The model under review builds one solid part; all positions refer to its coordinate system, in mm. Coordinates: 2 decimals unless noted, no trailing zeros. Loops run counter-clockwise (first coordinate to the right, second up) from the corner with the lowest first, then second, coordinate; pieces in that order, holes last. Notation, with made-up numbers: (30.25, 85.5) - (61.25, 85.5) arc R28 cw to (61.25, 108.5) - close; hole circle Ø8 at (14, 45.25). An arc over 180 degrees is marked (long way). One line per item, written item: value. Start each with the question number.
1. We need section C-C, the plane x = 15.5. Give the boundary of the cut face in (y, z), then the cut area to 3 significant figures.
2. To check wall thickness, follow line 1 (X direction, y = -15.5, z = -1.75); line 2 (Y direction, x = 15.5, z = -1.25); line 3 (X direction, y = 0, z = -3.2). State the ranges of each line that lie inside material, in increasing order.
3. We need section D-D, the plane z = -3. Give the boundary of the cut face in (x, y).
4. Insertion check: P1, Ø3.5, axis at x = -15.5, y = -15.5, coming from the +Z side. The pin has a flat end and moves straight along its axis. Give the tip position at first contact, or say it passes through.
5. We need section B-B, the plane x = 0. Give the boundary of the cut face in (y, z).
6. We need section A-A, the plane y = 15.5. Give the boundary of the cut face in (x, z).
7. Mouldability with a two-part tool opening along X and no side actions: class faces 1 (the face through (-17.483, -15.24, -2.535)), 2 (the face through (50, 0, -2)), 3 (the face through (-0.7, 11.5, -5)) as +X half, -X half, draft (parallel to the pull), parting line (faces both ways), or undercut.
Autodesk Inventor part; units mm, degrees
ref_plane "YZ Plane" through (0, 0, 0) normal (1, 0, 0) x (0, 1, 0)
ref_plane "XZ Plane" through (0, 0, 0) normal (0, 1, 0) x (-1, 0, 0)
ref_plane "XY Plane" through (0, 0, 0) normal (0, 0, 1) x (1, 0, 0)
sketch "Block1" plane through (0, 0, 0) normal (0, 0, 1) x (1, 0, 0)
  line L0 (-30.1, 34.1) -> (-9.9, 34.1)
  line L1 (-9.9, 34.1) -> (-9.9, 25.1)
  line L2 (-9.9, 25.1) -> (9.9, 25.1)
  line L3 (9.9, 25.1) -> (9.9, 34.1)
  line L4 (9.9, 34.1) -> (30.1, 34.1)
  line L5 (30.1, 34.1) -> (30.1, 25.1)
  line L6 (30.1, 25.1) -> (50.1, 25.1)
  line L7 (50.1, 25.1) -> (50.1, 16.5667)
  line L8 (50.1, 16.5667) -> (41.1, 16.5667)
  line L9 (41.1, 16.5667) -> (41.1, 6.7667)
  line L10 (41.1, 6.7667) -> (50.1, 6.7667)
  line L11 (50.1, 6.7667) -> (50.1, -6.7667)
  line L12 (50.1, -6.7667) -> (41.1, -6.7667)
  line L13 (41.1, -6.7667) -> (41.1, -16.5667)
  line L14 (41.1, -16.5667) -> (50.1, -16.5667)
  line L15 (50.1, -16.5667) -> (50.1, -25.1)
  line L16 (50.1, -25.1) -> (30.1, -25.1)
  line L17 (30.1, -25.1) -> (30.1, -34.1)
  line L18 (30.1, -34.1) -> (9.9, -34.1)
  line L19 (9.9, -34.1) -> (9.9, -25.1)
  line L20 (9.9, -25.1) -> (-9.9, -25.1)
  line L21 (-9.9, -25.1) -> (-9.9, -34.1)
  line L22 (-9.9, -34.1) -> (-30.1, -34.1)
  line L23 (-30.1, -34.1) -> (-30.1, -25.1)
  line L24 (-30.1, -25.1) -> (-50.1, -25.1)
  line L25 (-50.1, -25.1) -> (-50.1, -16.5667)
  line L26 (-50.1, -16.5667) -> (-41.1, -16.5667)
  line L27 (-41.1, -16.5667) -> (-41.1, -6.7667)
  line L28 (-41.1, -6.7667) -> (-50.1, -6.7667)
  line L29 (-50.1, -6.7667) -> (-50.1, 6.7667)
  line L30 (-50.1, 6.7667) -> (-41.1, 6.7667)
  line L31 (-41.1, 6.7667) -> (-41.1, 16.5667)
  line L32 (-41.1, 16.5667) -> (-50.1, 16.5667)
  line L33 (-50.1, 16.5667) -> (-50.1, 25.1)
  line L34 (-50.1, 25.1) -> (-30.1, 25.1)
  line L35 (-30.1, 25.1) -> (-30.1, 34.1)
  circle A0 centre (-30, 0) radius 4.6
  circle A1 centre (-15.5, 15.5) radius 2.1
  circle A2 centre (-15.5, -15.5) radius 2.1
  circle A3 centre (0, 0) radius 11.1
  circle A4 centre (15.5, 15.5) radius 2.1
  circle A5 centre (30, 0) radius 4.6
  circle A6 centre (15.5, -15.5) radius 2.1
  point P0 (0, 0)
sketch "Block2" plane through (0, 0, 0) normal (0, 0, 1) x (1, 0, 0)
  line L0 (9.8, 34.2) -> (30.2, 34.2)
  line L1 (30.2, 34.2) -> (30.2, 25.2)
  line L2 (30.2, 25.2) -> (50.2, 25.2)
  line L3 (50.2, 25.2) -> (50.2, 16.4667)
  line L4 (50.2, 16.4667) -> (41.2, 16.4667)
  line L5 (41.2, 16.4667) -> (41.2, 6.8667)
  line L6 (41.2, 6.8667) -> (50.2, 6.8667)
  line L7 (50.2, 6.8667) -> (50.2, -6.8667)
  line L8 (50.2, -6.8667) -> (41.2, -6.8667)
  line L9 (41.2, -6.8667) -> (41.2, -16.4667)
  line L10 (41.2, -16.4667) -> (50.2, -16.4667)
  line L11 (50.2, -16.4667) -> (50.2, -25.2)
  line L12 (50.2, -25.2) -> (30.2, -25.2)
  line L13 (30.2, -25.2) -> (30.2, -34.2)
  line L14 (30.2, -34.2) -> (9.8, -34.2)
  line L15 (9.8, -34.2) -> (9.8, -25.2)
  line L16 (9.8, -25.2) -> (-9.8, -25.2)
  line L17 (-9.8, -25.2) -> (-9.8, -34.2)
  line L18 (-9.8, -34.2) -> (-30.2, -34.2)
  line L19 (-30.2, -34.2) -> (-30.2, -25.2)
  line L20 (-30.2, -25.2) -> (-50.2, -25.2)
  line L21 (-50.2, -25.2) -> (-50.2, -16.4667)
  line L22 (-50.2, -16.4667) -> (-41.2, -16.4667)
  line L23 (-41.2, -16.4667) -> (-41.2, -6.8667)
  line L24 (-41.2, -6.8667) -> (-50.2, -6.8667)
  line L25 (-50.2, -6.8667) -> (-50.2, 6.8667)
  line L26 (-50.2, 6.8667) -> (-41.2, 6.8667)
  line L27 (-41.2, 6.8667) -> (-41.2, 16.4667)
  line L28 (-41.2, 16.4667) -> (-50.2, 16.4667)
  line L29 (-50.2, 16.4667) -> (-50.2, 25.2)
  line L30 (-50.2, 25.2) -> (-30.2, 25.2)
  line L31 (-30.2, 25.2) -> (-30.2, 34.2)
  line L32 (-30.2, 34.2) -> (-9.8, 34.2)
  line L33 (-9.8, 34.2) -> (-9.8, 25.2)
  line L34 (-9.8, 25.2) -> (9.8, 25.2)
  line L35 (9.8, 25.2) -> (9.8, 34.2)
  circle A0 centre (-15.5, 15.5) radius 2.2
  circle A1 centre (15.5, 15.5) radius 2.2
  circle A2 centre (30, 0) radius 4.7
  circle A3 centre (15.5, -15.5) radius 2.2
  circle A4 centre (-15.5, -15.5) radius 2.2
  circle A5 centre (-30, 0) radius 4.7
  circle A6 centre (0, 0) radius 11.2
  point P0 (0, 0)
sketch "Block3" plane through (0, 0, 0) normal (0, 0, 1) x (1, 0, 0)
  line L0 (9.9, 34.1) -> (30.1, 34.1)
  line L1 (30.1, 34.1) -> (30.1, 25.1)
  line L2 (30.1, 25.1) -> (50.1, 25.1)
  line L3 (50.1, 25.1) -> (50.1, 16.5667)
  line L4 (50.1, 16.5667) -> (41.1, 16.5667)
  line L5 (41.1, 16.5667) -> (41.1, 6.7667)
  line L6 (41.1, 6.7667) -> (50.1, 6.7667)
  line L7 (50.1, 6.7667) -> (50.1, -6.7667)
  line L8 (50.1, -6.7667) -> (41.1, -6.7667)
  line L9 (41.1, -6.7667) -> (41.1, -16.5667)
  line L10 (41.1, -16.5667) -> (50.1, -16.5667)
  line L11 (50.1, -16.5667) -> (50.1, -25.1)
  line L12 (50.1, -25.1) -> (30.1, -25.1)
  line L13 (30.1, -25.1) -> (30.1, -34.1)
  line L14 (30.1, -34.1) -> (9.9, -34.1)
  line L15 (9.9, -34.1) -> (9.9, -25.1)
  line L16 (9.9, -25.1) -> (-9.9, -25.1)
  line L17 (-9.9, -25.1) -> (-9.9, -34.1)
  line L18 (-9.9, -34.1) -> (-30.1, -34.1)
  line L19 (-30.1, -34.1) -> (-30.1, -25.1)
  line L20 (-30.1, -25.1) -> (-50.1, -25.1)
  line L21 (-50.1, -25.1) -> (-50.1, -16.5667)
  line L22 (-50.1, -16.5667) -> (-41.1, -16.5667)
  line L23 (-41.1, -16.5667) -> (-41.1, -6.7667)
  line L24 (-41.1, -6.7667) -> (-50.1, -6.7667)
  line L25 (-50.1, -6.7667) -> (-50.1, 6.7667)
  line L26 (-50.1, 6.7667) -> (-41.1, 6.7667)
  line L27 (-41.1, 6.7667) -> (-41.1, 16.5667)
  line L28 (-41.1, 16.5667) -> (-50.1, 16.5667)
  line L29 (-50.1, 16.5667) -> (-50.1, 25.1)
  line L30 (-50.1, 25.1) -> (-30.1, 25.1)
  line L31 (-30.1, 25.1) -> (-30.1, 34.1)
  line L32 (-30.1, 34.1) -> (-9.9, 34.1)
  line L33 (-9.9, 34.1) -> (-9.9, 25.1)
  line L34 (-9.9, 25.1) -> (9.9, 25.1)
  line L35 (9.9, 25.1) -> (9.9, 34.1)
  circle A0 centre (-15.5, 15.5) radius 2.1
  circle A1 centre (15.5, 15.5) radius 2.1
  circle A2 centre (30, 0) radius 4.6
  circle A3 centre (15.5, -15.5) radius 2.1
  circle A4 centre (-15.5, -15.5) radius 2.1
  circle A5 centre (-30, 0) radius 4.6
  circle A6 centre (0, 0) radius 11.1
  point P0 (0, 0)
sketch "Block4" plane through (0, 0, 0) normal (0, 0, 1) x (1, 0, 0)
  line L0 (-30.08, 30.58) -> (-9.92, 30.58)
  line L1 (-9.92, 30.58) -> (-9.92, 25.08)
  line L2 (-9.92, 25.08) -> (9.92, 25.08)
  line L3 (9.92, 25.08) -> (9.92, 30.58)
  line L4 (9.92, 30.58) -> (30.08, 30.58)
  line L5 (30.08, 30.58) -> (30.08, 25.08)
  line L6 (30.08, 25.08) -> (50.08, 25.08)
  line L7 (50.08, 25.08) -> (50.08, 16.5867)
  line L8 (50.08, 16.5867) -> (44.58, 16.5867)
  line L9 (44.58, 16.5867) -> (44.58, 6.7467)
  line L10 (44.58, 6.7467) -> (50.08, 6.7467)
  line L11 (50.08, 6.7467) -> (50.08, -6.7467)
  line L12 (50.08, -6.7467) -> (44.58, -6.7467)
  line L13 (44.58, -6.7467) -> (44.58, -16.5867)
  line L14 (44.58, -16.5867) -> (50.08, -16.5867)
  line L15 (50.08, -16.5867) -> (50.08, -25.08)
  line L16 (50.08, -25.08) -> (30.08, -25.08)
  line L17 (30.08, -25.08) -> (30.08, -30.58)
  line L18 (30.08, -30.58) -> (9.92, -30.58)
  line L19 (9.92, -30.58) -> (9.92, -25.08)
  line L20 (9.92, -25.08) -> (-9.92, -25.08)
  line L21 (-9.92, -25.08) -> (-9.92, -30.58)
  line L22 (-9.92, -30.58) -> (-30.08, -30.58)
  line L23 (-30.08, -30.58) -> (-30.08, -25.08)
  line L24 (-30.08, -25.08) -> (-50.08, -25.08)
  line L25 (-50.08, -25.08) -> (-50.08, -16.5867)
  line L26 (-50.08, -16.5867) -> (-44.58, -16.5867)
  line L27 (-44.58, -16.5867) -> (-44.58, -6.7467)
  line L28 (-44.58, -6.7467) -> (-50.08, -6.7467)
  line L29 (-50.08, -6.7467) -> (-50.08, 6.7467)
  line L30 (-50.08, 6.7467) -> (-44.58, 6.7467)
  line L31 (-44.58, 6.7467) -> (-44.58, 16.5867)
  line L32 (-44.58, 16.5867) -> (-50.08, 16.5867)
  line L33 (-50.08, 16.5867) -> (-50.08, 25.08)
  line L34 (-50.08, 25.08) -> (-30.08, 25.08)
  line L35 (-30.08, 25.08) -> (-30.08, 30.58)
  circle A0 centre (-30, 0) radius 4.88
  circle A1 centre (30, 0) radius 4.88
  circle A2 centre (15.5, 15.5) radius 2.08
  circle A3 centre (0, 0) radius 11.08
  circle A4 centre (-15.5, 15.5) radius 2.08
  circle A5 centre (-15.5, -15.5) radius 2.08
  circle A6 centre (15.5, -15.5) radius 2.08
  point P0 (0, 0)
sketch "Sketch10" plane through (0, 0, 0) normal (0, 0, 1) x (1, 0, 0)
  line L0 (50, -25) -> (-50, -25)
  line L1 (-50, -25) -> (-50, 25)
  line L2 (-50, 25) -> (50, 25)
  line L3 (50, 25) -> (50, -25)
  line L4 (50, -25) -> (-50, 25) construction
  line L5 (-50, -25) -> (50, 25) construction
  point P0 (0, 0)
  dimension "d21" = 100
  dimension "d22" = 50
extrude "Extrusion2" add sketch "Sketch10" against normal blind 5
sketch "Sketch13" plane through (0, 0, 0) normal (0, 0, 1) x (1, 0, 0)
  line L0 (0, -47.8822) -> (0, 48.5933)
  line L1 (-201.8331, 0) -> (92.0889, 0)
  point P0 (-15.5, 15.5)
  point P1 (15.5, 15.5)
  point P2 (-15.5, -15.5)
  point P3 (15.5, -15.5)
  dimension "d43" = 31
  dimension "d44" = 31
hole "Hole4" at (-15.5, 15.5, 0) at (15.5, 15.5, 0) at (-15.5, -15.5, 0) at (15.5, -15.5, 0) direction (0, 0, -1) diameter 4 end through all
sketch "Sketch16" plane through (0, 0, -5) normal (0, 0, -1) x (-1, 0, 0)
  line L0 (0, -47.8822) -> (0, 48.5933)
  point P0 (0, 0)
  point P1 (-30, 0)
  point P2 (30, 0)
  dimension "d52" = 60
hole "Hole5" at (30, 0, -5) at (-30, 0, -5) direction (0, 0, 1) diameter 5.2 end through all
sketch "Sketch17" plane through (0, 0, -5) normal (0, 0, -1) x (-1, 0, 0)
  point P0 (0, 0)
  point P1 (0, 0)
hole "Hole8" at (0, 0, -5) direction (0, 0, 1) diameter 22 end through all
sketch "Sketch33" plane through (0, 0, 0) normal (0, 0, 1) x (1, 0, 0)
  line L0 (-50, 25) -> (50, 25)
  line L1 (-50, -25) -> (-50, 25)
  line L2 (0, -47.8822) -> (0, 48.5933)
  line L3 (-201.8331, 0) -> (92.0889, 0)
  line L4 (-30, 25) -> (-10, 25)
  line L5 (-10, 25) -> (-10, 30.5)
  line L6 (-10, 30.5) -> (-30, 30.5)
  line L7 (-30, 30.5) -> (-30, 25)
  line L8 (30, 25) -> (10, 25)
  line L9 (10, 25) -> (10, 30.5)
  line L10 (10, 30.5) -> (30, 30.5)
  line L11 (30, 30.5) -> (30, 25)
  line L12 (-30, -25) -> (-10, -25)
  line L13 (-10, -25) -> (-10, -30.5)
  line L14 (-10, -30.5) -> (-30, -30.5)
  line L15 (-30, -30.5) -> (-30, -25)
  line L16 (10, -25) -> (10, -30.5)
  line L17 (30, -25) -> (10, -25)
  line L18 (10, -30.5) -> (30, -30.5)
  line L19 (30, -30.5) -> (30, -25)
  point P0 (-50, 16.6667)
  dimension "d121" = 20
  dimension "d122" = 5.5
  dimension "d123" = 20
extrude "Extrusion5" [suppressed]
sketch "Sketch34" plane through (0, 0, -5) normal (0, 0, -1) x (-1, 0, 0)
  line L0 (50, 25) -> (-50, 25)
  line L1 (-50, 25) -> (-50, -25)
  line L2 (-50, 16.6667) -> (-44.5, 16.6667)
  line L3 (-44.5, 16.6667) -> (-44.5, 6.6667)
  line L4 (-44.5, 6.6667) -> (-50, 6.6667)
  line L5 (-50, 6.6667) -> (-50, 16.6667)
  line L6 (201.8331, 0) -> (-92.0889, 0)
  line L7 (0, -47.8822) -> (0, 48.5933)
  line L8 (-50, -16.6667) -> (-44.5, -16.6667)
  line L9 (-44.5, -16.6667) -> (-44.5, -6.6667)
  line L10 (-44.5, -6.6667) -> (-50, -6.6667)
  line L11 (-50, -6.6667) -> (-50, -16.6667)
  line L12 (50, 16.6667) -> (44.5, 16.6667)
  line L13 (44.5, 16.6667) -> (44.5, 6.6667)
  line L14 (44.5, 6.6667) -> (50, 6.6667)
  line L15 (50, 6.6667) -> (50, 16.6667)
  line L16 (44.5, -16.6667) -> (44.5, -6.6667)
  line L17 (50, -16.6667) -> (44.5, -16.6667)
  line L18 (44.5, -6.6667) -> (50, -6.6667)
  line L19 (50, -6.6667) -> (50, -16.6667)
  point P0 (-30, 25)
  dimension "d131" = 5.5
  dimension "d132" = 10
  dimension "d133" = 8.3333
extrude "Extrusion6" [suppressed]
equation "\"d121\" = 0.2 * d21"
equation "\"d122\" = Wt"
equation "\"d123\" = 0.2 * d21"
equation "\"d129\" = Wt"
equation "\"d131\" = Wt"
equation "\"d132\" = 0.2 * d22"
equation "\"d133\" = 0.166667 * d22"
equation "\"d134\" = Wt"
properties part number "holder_plate" material "Wood (Birch)"
Findings below:
1. outline: (-25, -5) - (-17.5, -5) - (-17.5, 0) - (-25, 0) - close; (-13.5, -5) - (13.5, -5) - (13.5, 0) - (-13.5, 0) - close; (17.5, -5) - (25, -5) - (25, 0) - (17.5, 0) - close
1. area: 210 mm2
2. line 1: -50 to -17.5, -13.5 to 13.5, 17.5 to 50
2. line 2: -25 to -17.5, -13.5 to 13.5, 17.5 to 25
2. line 3: -50 to -32.6, -27.4 to -11, 11 to 27.4, 32.6 to 50
3. outline: (-50, -25) - (50, -25) - (50, 25) - (-50, 25) - close; hole circle Ø5.2 at (-30, 0); hole circle Ø4 at (-15.5, -15.5); hole circle Ø4 at (-15.5, 15.5); hole circle Ø22 at (0, 0); hole circle Ø4 at (15.5, -15.5); hole circle Ø4 at (15.5, 15.5); hole circle Ø5.2 at (30, 0)
4. P1: through
5. outline: (-25, -5) - (-11, -5) - (-11, 0) - (-25, 0) - close; (11, -5) - (25, -5) - (25, 0) - (11, 0) - close
6. outline: (-50, -5) - (-17.5, -5) - (-17.5, 0) - (-50, 0) - close; (-13.5, -5) - (13.5, -5) - (13.5, 0) - (-13.5, 0) - close; (17.5, -5) - (50, -5) - (50, 0) - (17.5, 0) - close
7. face 1: undercut
7. face 2: +X half
7. face 3: draft
